Source: CAD feature listing. Evaluate the final solid. Frame: model axes, mm. Coordinates: 2 decimals unless noted, no trailing zeros. Order: outer loops, then holes, each group sorted by start corner. A loop starts at its lowest first (then second) coordinate and runs counter-clockwise, first axis right, second up.
```python
from build123d import *
from build123d import SkipClean  # not in build123d's __all__

# Parameters (mm, degrees)
F1_DEPTH = 105.1
F3_DEPTH = 132.9


with BuildPart() as f1:
    # F0 (on Top) → F1 (new body)
    with BuildSketch(Plane.XY):
        with BuildLine():
            Line((-12.2990868875, 67.7678571429), (-1.7857142857, 9.83926951))
            ThreePointArc((-1.7857142857, 9.83926951), (-2.8810809532, -9.5759789338), (6.9184089901, 7.2204997781))
            Line((6.9184089901, 7.2204997781), (39.4409995563, 41.1631820199))
            ThreePointArc((39.4409995563, 41.1631820199), (44.9882549975, 55.6853190171), (38.4593810195, 69.7934128102))
            ThreePointArc((38.4593810195, 69.7934128102), (19.8153219741, 80.5054589403), (-1.6036428236, 82.3967064051))
            ThreePointArc((-1.6036428236, 82.3967064051), (-10.0907027029, 77.3775144162), (-12.2990868875, 67.7678571429))
        make_face()
    extrude(amount=F1_DEPTH)

    # F2 (on face) → F3 (join)
    with BuildSketch(Plane.XY):
        with BuildLine():
            ThreePointArc((-1.7857142857, 9.83926951), (-6.4086994446, -7.6764947358), (10, 0))
            ThreePointArc((10, 0), (9.197393378, 3.9252968104), (6.9184089901, 7.2204997781))
            ThreePointArc((6.9184089901, 7.2204997781), (2.8810809532, 9.5759789338), (-1.7857142857, 9.83926951))
        make_face()
    with SkipClean():  # cleaning this boolean's faces spoils the solid; the shape is the same uncleaned
        extrude(amount=-F3_DEPTH)


solid = f1.part
```
1. Material intervals for line 1 along Z through (x, y) = (-2, 72); line 2 along Y through (x, z) = (9, 19.5); line 3 along X through (y, z) = (-4, -28.5), sorted ascending.
2. Contact query for flat-ended pins moving along their axis: P1, Ø1.5, axis at y = 4, z = -38, coming from the +X side; P2, Ø10, axis at x = 25.5, z = 77.5, coming from the +Y side; P3, Ø6, axis at x = 4.5, z = -42, coming from the -Y side. Output: stop coordinate, or through.
3. Section query A-A, the plane z = 12. Output: boundary loops of the cut face in (x, y), plus the area to 3 significant figures.
4. Section query B-B, the plane x = 2.5. Output: boundary loops of the cut face in (y, z).
5. Draft query along Y for faces 1 (the flat face through (0, 0, -132.9)), 2 (the flat face through (-7.116, 39.209, 51.814)), 3 (the cylindrical face through (20.104, 80.414, 51.814)). Return one class per face: +Y half, -Y half, draft (parallel to the pull), parting line (faces both ways), or undercut.
6. Section query D-D, the plane z = -26. Output: boundary loops of the cut face in (x, y), plus the area to 3 significant figures.
7. Section query C-C, the plane y = 20. Output: boundary loops of the cut face in (x, z), plus the area to 3 significant figures.
Answer key:
1. line 1: z = 0 to 105.1
1. line 2: y = -4.36 to 4.36, 9.39 to 82.63
1. line 3: x = -9.17 to 9.17
2. P1: stops at x = 9.46
2. P2: stops at y = 80.28
2. P3: stops at y = -9.89
3. outline: (-12.3, 67.77) - (-1.79, 9.84) arc R10 ccw (long way) to (6.92, 7.22) - (39.44, 41.16) arc R20 ccw to (38.46, 69.79) arc R50 ccw to (-1.6, 82.4) arc R12.5 ccw to start
3. area: 3,240 mm2
4. outline: (-9.68, -132.9) - (9.68, -132.9) - (9.68, 0) - (82.76, 0) - (82.76, 105.1) - (-9.68, 105.1) - close
5. face 1: draft
5. face 2: undercut
5. face 3: +Y half
6. outline: circle Ø20 at (0, 0)
6. area: 314 mm2
7. outline: (-3.63, 0) - (19.16, 0) - (19.16, 105.1) - (-3.63, 105.1) - close
7. area: 2,400 mm2
